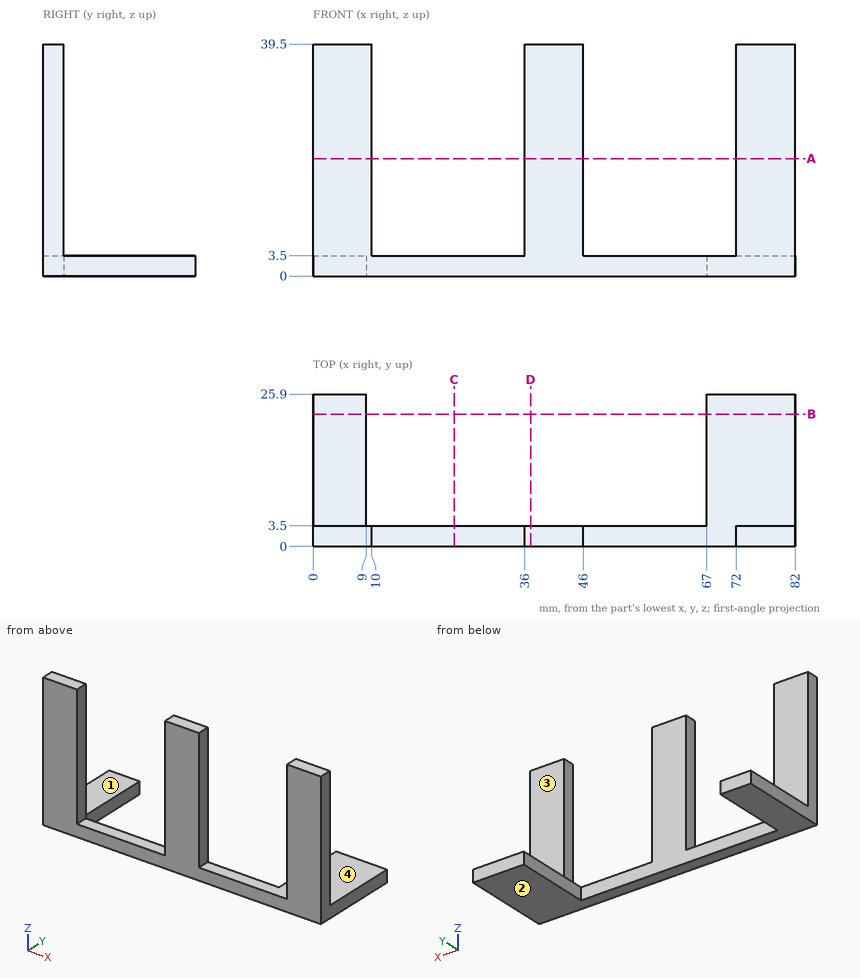
For this review, use the dimensioned drawing (mm, ordinates from the lowest corner) and the shaded views. A direction names the side the tool comes from. Give positions to 0.01 mm unless a question says otherwise; leave off trailing zeros. Order: outer loops, then holes, each group sorted by start corner. A loop starts at its lowest first (then second) coordinate and runs counter-clockwise, first axis right, second up. Notation, with made-up numbers: (16.5, -39) -> (40.5, -39) arc R8 ccw to (40.5, -33) -> close; hole circle Ø10 at (50.25, 62). An arc over 180 degrees is marked (long way). Write item = value, one per line. Start each with the question number.
(1) Take a section at C-C (x = 24). Write out the cut boundary in (y, z), plus the area to 4 significant figures.
(2) For L1, parallel to X at y = 2, z = 30; L2, parallel to Y at x = 40.5, z = 34, list the stretches that pass through material, from the lowest coordinate up. Write a range as from..to.
(3) Draft analysis for pull direction X (two halves, no side actions). For the marked faces 3 and 4, state which applies: +X half, -X half, draft (parallel to the pull), parting line (faces both ways), or undercut.
(4) Tool access review of the marked faces 1 and 2: name each direction out of +Z, -Z, +X, -X, +Y, -Y from which nothing blocks a thin tool from reaching the whole face with its end or side.
(5) Take a section at D-D (x = 37). Write out the cut boundary in (y, z).
(6) Take a section at A-A (z = 20). Write out the cut boundary in (x, y), plus the area to 3 significant figures.
(7) For pin 1 Ø10 at (x, z) = (72.5, 14.5) entering from +Y; pin 2 Ø4.5 at (x, y) = (6, 18.5) entering from +Z, all flat-tipped, find the tip position at first contact; note any pin that passes through.
(8) Take a section at B-B (y = 22.5). Write out the cut boundary in (x, z), plus the area to 3 significant figures.
Returned:
q1.outline = (0, 0) -> (3.5, 0) -> (3.5, 3.5) -> (0, 3.5) -> close
q1.area = 12.25 mm²
q2.L1 = 0..10, 36..46, 72..82
q2.L2 = 0..3.5
q3.face_3 = draft
q3.face_4 = undercut
q4.face_1 = +Z, +X, -X, +Y
q4.face_2 = -Z, +X, -X, +Y, -Y
q5.outline = (0, 0) -> (3.5, 0) -> (3.5, 39.5) -> (0, 39.5) -> close
q6.outline = (0, 0) -> (10, 0) -> (10, 3.5) -> (0, 3.5) -> close; (36, 0) -> (46, 0) -> (46, 3.5) -> (36, 3.5) -> close; (72, 0) -> (82, 0) -> (82, 3.5) -> (72, 3.5) -> close
q6.area = 105 mm²
q7.pin_1 = 3.5
q7.pin_2 = 3.5
q8.outline = (0, 0) -> (9, 0) -> (9, 3.5) -> (0, 3.5) -> close; (67, 0) -> (82, 0) -> (82, 3.5) -> (67, 3.5) -> close
q8.area = 84.0 mm²
